The listing builds one solid part. Answer for the finished solid, in the listing's coordinates (mm). Coordinates: 2 decimals unless noted, no trailing zeros. Order: outer loops, then holes, each group sorted by start corner. A loop starts at its lowest first (then second) coordinate and runs counter-clockwise, first axis right, second up. Notation, with made-up numbers: (75.5, 71.25) -> (126.5, 71.25) arc R21 ccw to (126.5, 87.25) -> close; hole circle Ø7 at (-9, 77). An arc over 180 degrees is marked (long way). Answer in a Markdown table with one row per item.
```python
from build123d import *

# Parameters (mm, degrees)
CROQUIS1_W              = 70
CROQUIS1_H              = 50
SALIENTE_EXTRUIR1_DEPTH = 1
CROQUIS2_R              = 1.5
CORTAR_EXTRUIR1_DEPTH   = 1


with BuildPart() as part:
    # Croquis1 → Saliente-Extruir1 (new body)
    with BuildSketch(Plane.XY):
        Rectangle(CROQUIS1_W, CROQUIS1_H)
    extrude(amount=SALIENTE_EXTRUIR1_DEPTH)

    # Croquis2 → Cortar-Extruir1 (cut)
    with BuildSketch(Plane(origin=(0, 0, 0), x_dir=(-1, 0, 0), z_dir=(0, 0, -1))):
        with Locations((-25, 0)):
            Circle(CROQUIS2_R)
        Circle(CROQUIS2_R)
        with Locations((25, 0)):
            Circle(CROQUIS2_R)
    extrude(amount=-CORTAR_EXTRUIR1_DEPTH, mode=Mode.SUBTRACT)


solid = part.part
```
(1) A cutting plane is placed at A-A, the plane y = 0. Determine the outline of the cut face in (x, z), then the cut area to 3 significant figures.
Check values:
| item | result |
|---|---|
| outline | (-35, 0) -> (-26.5, 0) -> (-26.5, 1) -> (-35, 1) -> close; (-23.5, 0) -> (-1.5, 0) -> (-1.5, 1) -> (-23.5, 1) -> close; (1.5, 0) -> (23.5, 0) -> (23.5, 1) -> (1.5, 1) -> close; (26.5, 0) -> (35, 0) -> (35, 1) -> (26.5, 1) -> close |
| area | 61.0 mm² |
(2) A cutting plane is placed at B-B, the plane x = -25. Determine the outline of the cut face in (y, z), then the cut area to 3 significant figures.
Check values:
| item | result |
|---|---|
| outline | (-25, 0) -> (-1.5, 0) -> (-1.5, 1) -> (-25, 1) -> close; (1.5, 0) -> (25, 0) -> (25, 1) -> (1.5, 1) -> close |
| area | 47.0 mm² |
(3) Find the intervals of material crossed by line 1 along Y through (x, z) = (0, 0.35); line 2 along Y through (x, z) = (-25.5, 0.6), in increasing order. Write a range as from..to.
Check values:
| item | result |
|---|---|
| line 1 | -25..-1.5, 1.5..25 |
| line 2 | -25..-1.41, 1.41..25 |
(4) A flat-ended cylindrical pin translates along its axis: pin 1 (1.8 mm diameter, centred on x = 0, y = 0, fed in from +Z). Find the tip coordinate at first contact, or state that the pin passes through.
Check values:
| item | result |
|---|---|
| pin 1 | through |
(5) For a pull along Y with two mould halves and no side action, classify faces 1 (the cylindrical face through (-23.5, 0.07, 0.49)), 2 (the flat face through (0, 6, 0)) as released by +Y, released by -Y, zero draft, split by the parting line, or undercut.
Check values:
| item | result |
|---|---|
| face 1 | undercut |
| face 2 | zero draft |
